from build123d import *

# Parameters (mm, degrees)
SKETCH1_R                               = 47.5
BOSS_EXTRUDE1_DEPTH                     = 20
SKETCH2_R                               = 19.9
BOSS_EXTRUDE2_DEPTH                     = 65
SKETCH3_R                               = 30
BOSS_EXTRUDE3_DEPTH                     = 30
SKETCH4_R                               = 19.9
BOSS_EXTRUDE4_DEPTH                     = 140
BOSS_EXTRUDE5_DEPTH                     = 30
BOSS_EXTRUDE5_DEPTH_BACK                = 30
CUT_EXTRUDE1_DEPTH                      = 40
SKETCH7_R                               = 7.5
CUT_EXTRUDE2_DEPTH                      = 78.5
SKETCH8_R                               = 20
CUT_EXTRUDE3_DEPTH                      = 15
CBORE_FOR_M5_HEX_HEAD_BOLT3_D           = 10
CBORE_FOR_M5_HEX_HEAD_BOLT3_CBORE_D     = 14
CBORE_FOR_M5_HEX_HEAD_BOLT3_CBORE_DEPTH = 10
CIRPATTERN1_COUNT                       = 4


with BuildPart() as part:
    # Sketch1 → Boss-Extrude1 (new body)
    with BuildSketch(Plane(origin=(0, 0, 0), x_dir=(1, 0, 0), z_dir=(0, 1, 0))):
        Circle(SKETCH1_R)
    extrude(amount=BOSS_EXTRUDE1_DEPTH)

    # Sketch2 → Boss-Extrude2 (add)
    with BuildSketch(Plane(origin=(0, 20, 0), x_dir=(1, 0, 0), z_dir=(0, 1, 0))):
        Circle(SKETCH2_R)
    extrude(amount=BOSS_EXTRUDE2_DEPTH)

    # Sketch3 → Boss-Extrude3 (add)
    with BuildSketch(Plane(origin=(0, 85, 0), x_dir=(1, 0, 0), z_dir=(0, 1, 0))):
        Circle(SKETCH3_R)
    extrude(amount=BOSS_EXTRUDE3_DEPTH)

    # Sketch4 → Boss-Extrude4 (add)
    with BuildSketch(Plane(origin=(0, 115, 0), x_dir=(1, 0, 0), z_dir=(0, 1, 0))):
        Circle(SKETCH4_R)
    extrude(amount=BOSS_EXTRUDE4_DEPTH)

    # Sketch5 → Boss-Extrude5 (add, two sides)
    with BuildSketch(Plane.XY) as boss_extrude5_sk:
        with BuildLine():
            Line((-4.684895629, 115), (60, 115))
            ThreePointArc((60, 115), (71.456034828, 106.572011481), (66.820181321, 93.126544336))
            Line((66.820181321, 93.126544336), (54.485559633, 84.606289695))
            Line((54.485559633, 84.606289695), (-4.684895629, 85))
            Line((-4.684895629, 85), (-4.684895629, 115))
        make_face()
    extrude(amount=BOSS_EXTRUDE5_DEPTH)
    extrude(boss_extrude5_sk.sketch, amount=-BOSS_EXTRUDE5_DEPTH_BACK)

    # Sketch6 → Cut-Extrude1 (cut)
    with BuildSketch(Plane(origin=(0, 115, 0), x_dir=(1, 0, 0), z_dir=(0, 1, 0))):
        with BuildLine():
            Line((85.613181264, 20), (85.613181264, -20))
            Line((85.613181264, -20), (22.360679775, -20))
            ThreePointArc((22.360679775, -20), (30, 0), (22.360679775, 20))
            Line((22.360679775, 20), (85.613181264, 20))
        make_face()
    extrude(amount=-CUT_EXTRUDE1_DEPTH, mode=Mode.SUBTRACT)

    # Sketch7 → Cut-Extrude2 (cut, through all)
    with BuildSketch(Plane.XY.offset(30)):
        with Locations((55, 103)):
            Circle(SKETCH7_R)
    extrude(amount=-CUT_EXTRUDE2_DEPTH, mode=Mode.SUBTRACT)

    # Sketch8 → Cut-Extrude3 (cut)
    with BuildSketch(Plane.XZ):
        Circle(SKETCH8_R)
    extrude(amount=-CUT_EXTRUDE3_DEPTH, mode=Mode.SUBTRACT)

    # CBORE for M5 Hex Head Bolt3 (through all)
    with Locations(Plane(origin=(0, 20, 0), x_dir=(1, 0, 0), z_dir=(0, 1, 0))):
        with Locations((0, 38)):
            cbore_for_m5_hex_head_bolt3 = CounterBoreHole(CBORE_FOR_M5_HEX_HEAD_BOLT3_D / 2, CBORE_FOR_M5_HEX_HEAD_BOLT3_CBORE_D / 2, CBORE_FOR_M5_HEX_HEAD_BOLT3_CBORE_DEPTH)

    # CirPattern1: CBORE for M5 Hex Head Bolt3 ×4 about axis
    cirpattern1_axis = Axis((0, 0, 0), (0, 1, 0))
    for i in range(1, CIRPATTERN1_COUNT):
        add(cbore_for_m5_hex_head_bolt3.rotate(cirpattern1_axis, i * 360 / CIRPATTERN1_COUNT), mode=Mode.SUBTRACT)


solid = part.part
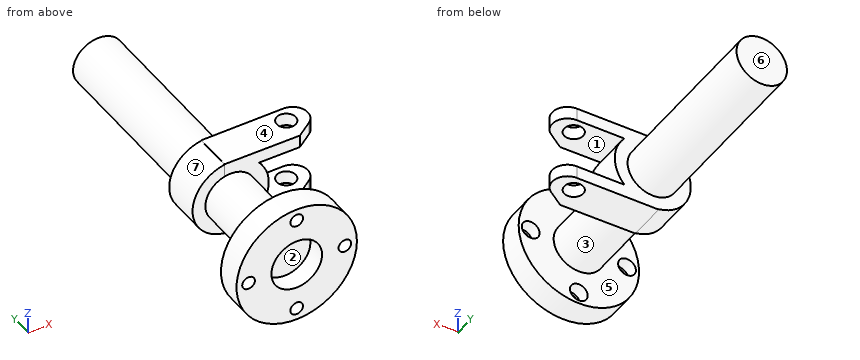
Build history of the part. All positions in model axes, mm. Face numbers are marked on the shaded views. A direction names the side the tool comes from. Round coordinates to 2 decimals unless told otherwise and drop trailing zeros. Write each loop counter-clockwise with the first axis right and the second up, starting at its lowest first coordinate (ties: lowest second). Pieces come first, ordered by that corner, then holes. Notation, with made-up numbers: (19.25, -6) - (35.25, -6) arc R6 ccw to (35.25, 4) - close; hole circle Ø7 at (-18, 77). An arc over 180 degrees is marked (long way). One line per question, with ' | ' between items.
1. Drill centre lines: line 1 along Z through (x, y) = (0, 5.5); line 2 along Z through (x, y) = (0, 11.5); line 3 along X through (y, z) = (18, 0). Where is each one in solid material? Low to high. Write a range as from..to.
Results are:
line 1: -47.5..-43, -33..-20, 20..33, 43..47.5 | line 2: -47.5..-45, -31..-20, 20..31, 45..47.5 | line 3: -47.5..-45, -31..31, 45..47.5
2. Band-saw the part on A-A, the plane z = -38. Write the cut outline in (x, y), and give its area (3 significant figures).
Results are:
outline: (-28.5, 0) - (-5, 0) - (-5, 10) - (-7, 10) - (-7, 20) - (-28.5, 20) - close; (5, 0) - (28.5, 0) - (28.5, 20) - (7, 20) - (7, 10) - (5, 10) - close | area: 900 mm^2
3. Mould opens along Y. For the marked faces 5, 6 and 7 say: released by +Y, released by -Y, zero draft, split by the parting line, or undercut.
Results are:
face 5: undercut | face 6: released by +Y | face 7: zero draft
4. Drop flat-ended pins along their axis: pin 1 Ø8 at (y, z) = (128, -10.5) entering from -X; pin 2 Ø3 at (y, z) = (223, -11) entering from +X; pin 3 Ø8 at (y, z) = (92, 7) entering from +X. Give the stop position or say it passes through.
Results are:
pin 1: x = -18.81 | pin 2: x = 17.49 | pin 3: x = 29.85
5. Band-saw the part on C-C, the plane x = -38. Write the cut outline in (y, z).
Results are:
outline: (0, -28.5) - (20, -28.5) - (20, -7) - (10, -7) - (10, -5) - (0, -5) - close; (0, 5) - (10, 5) - (10, 7) - (20, 7) - (20, 28.5) - (0, 28.5) - close
6. Tool access for the marked faces 1, 2, 3 and 4: list every direction of +Z, -Z, +X, -X, +Y, -Y with a clear straight run to the whole face (end or side of a thin tool).
Results are:
face 1: +X, +Y | face 2: -Y | face 3: none | face 4: +Z, +X, -X, +Y
7. Band-saw the part on B-B, the plane y = 103. Write the cut outline in (x, z), and give its area (3 significant figures).
Results are:
outline: (-4.68, -30) - (47.5, -30) - (47.5, -20) - (22.36, -20) arc R30 ccw to (22.36, 20) - (47.5, 20) - (47.5, 30) - (-4.68, 30) - (-4.68, 29.63) arc R30 ccw to (-4.68, -29.63) - close; (62.5, -30) - (72, -30) - (72, -20) - (62.5, -20) - close; (62.5, 20) - (72, 20) - (72, 30) - (62.5, 30) - close | area: 3,660 mm^2
8. Band-saw the part on D-D, the plane x = 38. Write the cut outline in (y, z), and give its area (3 significant figures).
Results are:
outline: (0, -28.5) - (20, -28.5) - (20, -7) - (10, -7) - (10, -5) - (0, -5) - close; (0, 5) - (10, 5) - (10, 7) - (20, 7) - (20, 28.5) - (0, 28.5) - close; (84.72, -30) - (115, -30) - (115, -20) - (84.72, -20) - close; (84.72, 20) - (115, 20) - (115, 30) - (84.72, 30) - close | area: 1,510 mm^2
